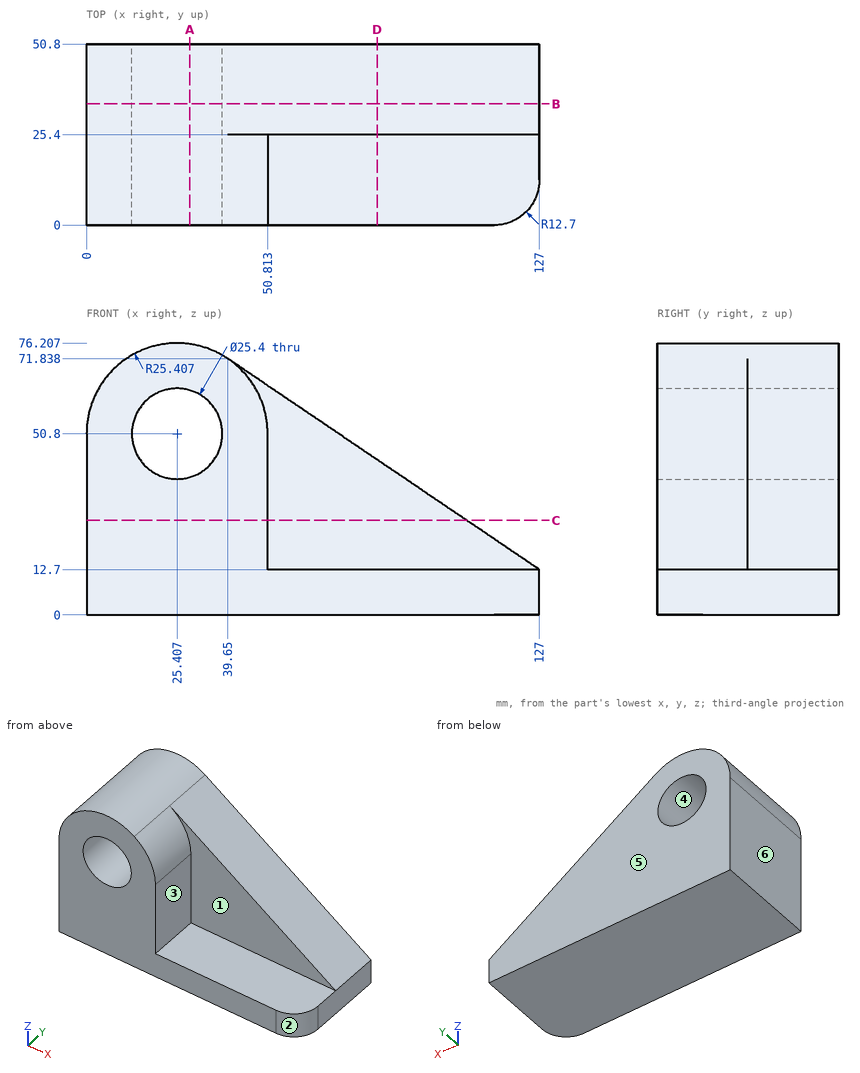
Study the drawing (mm; zero at the part's minimum x, y, z) and answer. A direction names the side the tool comes from. Round coordinates to 2 decimals unless told otherwise and drop trailing zeros. Write each loop counter-clockwise with the first axis right and the second up, starting at its lowest first coordinate (ties: lowest second). Pieces come first, ordered by that corner, then holes. Notation, with made-up numbers: (33, -17) - (39, -17) arc R17 cw to (39, -1) - close; hole circle Ø5 at (29, 49). An arc over 180 degrees is marked (long way). Return JSON: item names as keys, results as strings. Group by question number.
Q1. For the marked faces 1 and 2, determine the directions among +Z, -Z, +X, -X, +Y, -Y from which every point of the face is accessible in a straight line to the end or side of a thin tool.
Q2. Find the intervals of material crossed by L1, parallel to Y at x = 95, z = 23; L2, parallel to Z at x = 30.5, y = 46.5 (1 decimal); L3, parallel to Z at x = 77, y = 4.5, in increasing order.
Q3. The part is cut by section C-C on z = 26.5. Write down the section's boundary in (x, y).
Q4. The part is cut by section A-A on x = 29. Write down the section's boundary in (y, z).
Q5. The part is cut by section B-B on y = 34. Write down the section's boundary in (x, z).
Q6. The mould has two halves that part along X. Classify the marked faces 3, 4, 5 and 6: released by +X, released by -X, zero draft, split by the parting line, or undercut.
Q7. The part is cut by section D-D on x = 81.5. Write down the section's boundary in (y, z) (1 decimal), then the cut area to 3 significant figures.
Q8. Each of these flat-tipped pins is pushed along its axis until it touches: pin 1 Ø2 at (y, z) = (17.5, 67) entering from -X; pin 2 Ø6 at (y, z) = (8.5, 42.5) entering from +X; pin 3 Ø3 at (y, z) = (18.5, 55.5) entering from -X. Where does it stop, or does it pass through?
Solved:
{
 "1": {"face 1": "+Z, +X, -Y", "face 2": "+Z, -Z, +X, -Y"},
 "2": {"L1": "25.4 to 50.8", "L2": "0 to 39.2, 62.4 to 75.7", "L3": "0 to 12.7"},
 "3": {"outline": "(0, 0) - (50.81, 0) - (50.81, 25.4) - (106.62, 25.4) - (106.62, 50.8) - (0, 50.8) - close"},
 "4": {"outline": "(0, 0) - (50.8, 0) - (50.8, 38.62) - (0, 38.62) - close; (0, 62.98) - (50.8, 62.98) - (50.8, 75.95) - (0, 75.95) - close"},
 "5": {"outline": "(0, 0) - (127, 0) - (127, 12.7) - (39.65, 71.84) arc R25.41 ccw to (0, 50.8) - close; hole circle Ø25.4 at (25.41, 50.8)"},
 "6": {"face 3": "released by +X", "face 4": "undercut", "face 5": "zero draft", "face 6": "released by -X"},
 "7": {"outline": "(0, 0) - (50.8, 0) - (50.8, 43.5) - (25.4, 43.5) - (25.4, 12.7) - (0, 12.7) - close", "area": "1,430 mm²"},
 "8": {"pin 1": "x = 5.05", "pin 2": "x = 50.81", "pin 3": "x = 0.2"}
}
